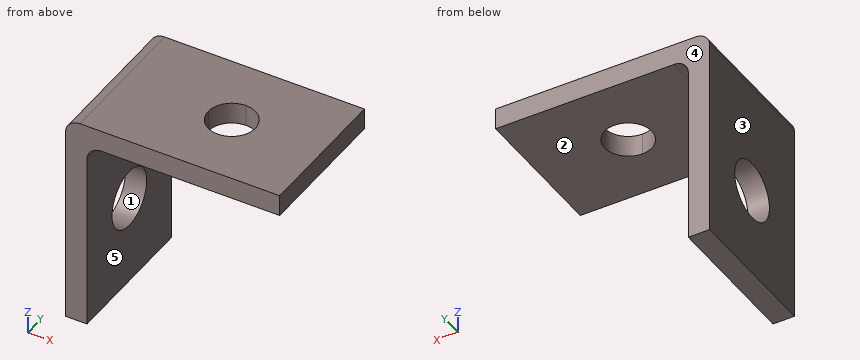
```python
from build123d import *

# Parameters (mm, degrees)
EXTRUDE_1_DEPTH     = 10
CUT_EXTRUDE_3_DEPTH = 8
SKETCH_12_R         = 2.05
CUT_EXTRUDE_5_DEPTH = 95


with BuildPart() as part:
    # Эскиз1 → Бобышка-Вытянуть1 (new body)
    with BuildSketch(Plane(origin=(0, 0, 0), x_dir=(1, 0, 0), z_dir=(0, 1, 0))):
        with BuildLine():
            Line((0, 1), (0, 15))
            Line((0, 15), (1.5, 15))
            Line((1.5, 15), (1.5, 2.5))
            ThreePointArc((1.5, 2.5), (1.792893219, 1.792893219), (2.5, 1.5))
            Line((2.5, 1.5), (15, 1.5))
            Line((15, 1.5), (15, 0))
            Line((15, 0), (1, 0))
            ThreePointArc((1, 0), (0.292893219, 0.292893219), (0, 1))
        make_face()
    extrude(amount=EXTRUDE_1_DEPTH)

    # Эскиз6 → Вырез-Вытянуть3 (cut)
    with BuildSketch(Plane(origin=(-307.940790238, -349.204468703, -1.5), x_dir=(-0.9998892265297747, 0.014884040771535371, 0), z_dir=(0, 0, -1))):
        with BuildLine():
            ThreePointArc((-309.659295343, 358.877763083), (-310.142569154, 360.044489272), (-311.309295343, 360.527763083))
            Line((-311.309295343, 360.527763083), (-311.309295343, 357.227763083))
            ThreePointArc((-311.309295343, 357.227763083), (-310.142569154, 357.711036894), (-309.659295343, 358.877763083))
        make_face()
        with BuildLine():
            Line((-311.309295343, 357.227763083), (-311.309295343, 360.527763083))
            ThreePointArc((-311.309295343, 360.527763083), (-312.959295343, 358.877763083), (-311.309295343, 357.227763083))
        make_face()
    extrude(amount=-CUT_EXTRUDE_3_DEPTH, mode=Mode.SUBTRACT)

    # Эскиз12 → Вырез-Вытянуть5 (cut)
    with BuildSketch(Plane(origin=(1.5, 0, 0), x_dir=(0, 0, -1), z_dir=(1, 0, 0))):
        with Locations((8.75, 5)):
            Circle(SKETCH_12_R)
    extrude(amount=-CUT_EXTRUDE_5_DEPTH, mode=Mode.SUBTRACT)


solid = part.part
```
Part model, mm, in its own coordinate system. Face numbers are marked on the shaded views. A direction names the side the tool comes from. Give positions to 0.01 mm unless a question says otherwise; leave off trailing zeros. Order: outer loops, then holes, each group sorted by start corner. A loop starts at its lowest first (then second) coordinate and runs counter-clockwise, first axis right, second up. Notation, with made-up numbers: M -2.75,-38.75 L 52.25,-38.75 A21 ccw 52.25,-17.75 Z; hole C -22.75,-37 d9. An arc over 180 degrees is marked long. Use a Markdown table: item, result. Add a question column.
(1) Saw through at A-A, the plane z = -8.75. Give the cut face in (x, y).
(2) Saw through at C-C, the plane z = -1.25. Give the cut face in (x, y), and give its area (3 significant figures).
(3) Probe line 1 along Y through (x, z) = (0.9, -8.75); line 2 along X through (y, z) = (7, -13); line 3 along Z through (x, y) = (13.5, 3.5). List the from-to ranges inside material, lowest first. Write a range as [from, to].
(4) Drop flat-ended pins along their axis: P1, Ø1.5, axis at y = 5, z = -4, coming from the +X side; P2, Ø3, axis at x = 8, y = 5, coming from the -Z side. Give the stop position or say it passes through.
(5) Saw through at B-B, the plane x = 9.75. Give the cut face in (y, z), and give its area (3 significant figures).
(6) Mould opens along Z. For the marked faces 1, 2 and 3 say: +Z half, -Z half, draft (parallel to the pull), parting line (faces both ways), or undercut.
(7) Saw through at D-D, the plane x = 6.5. Give the cut face in (y, z).
(8) 3-axis set-ups, long thin cutter, end or side, ignore diameter. For the marked faces 4 and 5: which of +Z, -Z, +X, -X, +Y, -Y reach the whole face in a straight line?
Answer key:
| question | item | result |
|---|---|---|
| 1 | outline | M 0,0 L 1.5,0 L 1.5,2.95 L 0,2.95 Z; M 0,7.05 L 1.5,7.05 L 1.5,10 L 0,10 Z |
| 2 | outline | M 0,0 L 15,0 L 15,10 L 0,10 Z; hole C 8.68,5 d3.3 |
| 2 | area | 141 mm^2 |
| 3 | line 1 | [0, 2.95], [7.05, 10] |
| 3 | line 2 | [0, 1.5] |
| 3 | line 3 | [-1.5, 0] |
| 4 | P1 | x = 1.5 |
| 4 | P2 | z = -1.5 |
| 5 | outline | M 0,-1.5 L 3.75,-1.5 L 3.75,0 L 0,0 Z; M 6.25,-1.5 L 10,-1.5 L 10,0 L 6.25,0 Z |
| 5 | area | 11.2 mm^2 |
| 6 | face 1 | undercut |
| 6 | face 2 | -Z half |
| 6 | face 3 | draft |
| 7 | outline | M 0,-1.5 L 10,-1.5 L 10,0 L 0,0 Z |
| 8 | face 4 | +Z, -Z, +X, -X, +Y |
| 8 | face 5 | -Z, +X, +Y, -Y |
